Source: CAD feature listing. Evaluate the final solid. Frame: model axes, mm. A direction names the side the tool comes from. Give positions to 0.01 mm unless a question says otherwise; leave off trailing zeros. Order: outer loops, then holes, each group sorted by start corner. A loop starts at its lowest first (then second) coordinate and runs counter-clockwise, first axis right, second up.
from build123d import *

# Parameters (mm, degrees)
SKETCH1_W                = 58.5
SKETCH1_H                = 75
SKETCH1_R                = 8
SKETCH1_R_2              = 1.5
BOSS_EXTRUDE1_DEPTH      = 2.5
SKETCH4_W                = 58.5
SKETCH4_H                = 40
BOSS_EXTRUDE2_DEPTH      = 7.5
M3_CLEARANCE_HOLE1_D     = 3.2
M3_CLEARANCE_HOLE1_DEPTH = 4
M3_CLEARANCE_HOLE1_TIP   = 0.96137699
FILLET1_R                = 10
FILLET2_R                = 7.5


with BuildPart() as part:
    # Sketch1 → Boss-Extrude1 (new, symmetric)
    with BuildSketch(Plane.XY):
        with Locations((-9.25, 23)):
            Rectangle(SKETCH1_W, SKETCH1_H)
        Circle(SKETCH1_R, mode=Mode.SUBTRACT)
        with Locations((-24, -9)):
            Circle(SKETCH1_R_2, mode=Mode.SUBTRACT)
        with Locations((9, -9)):
            Circle(SKETCH1_R_2, mode=Mode.SUBTRACT)
        with Locations((9, 9)):
            Circle(SKETCH1_R_2, mode=Mode.SUBTRACT)
        with Locations((-24, 9)):
            Circle(SKETCH1_R_2, mode=Mode.SUBTRACT)
    extrude(amount=BOSS_EXTRUDE1_DEPTH, both=True)

    # Sketch4 → Boss-Extrude2 (add)
    with BuildSketch(Plane(origin=(0, 0, -2.5), x_dir=(-1, 0, 0), z_dir=(0, 0, -1))):
        with Locations((9.25, 40.5)):
            Rectangle(SKETCH4_W, SKETCH4_H)
    extrude(amount=BOSS_EXTRUDE2_DEPTH)

    # M3 Clearance Hole1
    with Locations(Plane(origin=(0, 60.5, 0), x_dir=(1, 0, 0), z_dir=(0, 1, 0))):
        with Locations((-31.95, 3), (11.75, 3)):
            Hole(M3_CLEARANCE_HOLE1_D / 2, depth=M3_CLEARANCE_HOLE1_DEPTH)
            with Locations((0, 0, -(M3_CLEARANCE_HOLE1_DEPTH + M3_CLEARANCE_HOLE1_TIP / 2))):  # 118° drill point
                Cone(0, M3_CLEARANCE_HOLE1_D / 2, M3_CLEARANCE_HOLE1_TIP, mode=Mode.SUBTRACT)

    # Fillet1
    fillet1_edges = [part.edges().sort_by_distance(p)[0] for p in [
        (20, -14.5, 0),
        (-38.5, -14.5, 0),
    ]]
    fillet(fillet1_edges, radius=FILLET1_R)

    # Fillet2
    fillet2_edges = [part.edges().sort_by_distance(p)[0] for p in [
        (-38.5, 40.5, -10),
        (20, 40.5, -10),
    ]]
    fillet(fillet2_edges, radius=FILLET2_R)


solid = part.part
1) Reachability of faces 1 (the face through (-9, 20.5, -6)), 2 (the face through (-9, 60.5, -4)), 3 (the face through (-30.35, 58.47, -3.07)) from +Z, -Z, +X, -X, +Y, -Y: full face, straight path, thin tool, end or side. Return the list, or none.
Checks:
face 1: -Z, +X, -X, -Y
face 2: +Z, -Z, +X, -X, +Y
face 3: +Y
2) Section query D-D on z = 0.5. Output: boundary loops of the cut face in (x, y), and give its area (3 significant figures).
Checks:
outline: (-38.5, -4.5) arc R10 ccw to (-28.5, -14.5) - (10, -14.5) arc R10 ccw to (20, -4.5) - (20, 60.5) - (-38.5, 60.5) - close; hole circle Ø3 at (-24, -9); hole circle Ø3 at (-24, 9); hole circle Ø16 at (0, 0); hole circle Ø3 at (9, -9); hole circle Ø3 at (9, 9)
area: 4,120 mm2
3) First-contact query: pin 1 Ø4 at (x, y) = (-11, 4) entering from -Z; pin 2 Ø4 at (x, z) = (-20.5, -6.5) entering from -Y; pin 3 Ø2 at (y, z) = (31, -7.5) entering from -X. Flat tips, straight axial feed; report the tip coordinate or a pass-through.
Checks:
pin 1: stops at z = -2.5
pin 2: stops at y = 20.5
pin 3: stops at x = -37.34
4) Pull-direction query (X, two-part tool) for faces 4 (the face through (-36.245, 40.78, -7.861)), 5 (the face through (-10, 3, -2.5)), 6 (the face through (11.529, 55.706, -2.831)), 7 (the face through (-25.2, 8.1, 0)); classes: +X half, -X half, draft (parallel to the pull), parting line (faces both ways), or undercut.
Checks:
face 4: -X half
face 5: draft
face 6: undercut
face 7: undercut
5) Ray query, L1, parallel to Y at x = 9, z = -0.4; L2, parallel to Y at x = 0, z = -1.4; L3, parallel to Y at x = 5.5, z = -6.75. Return the intervals inside material, ascending.
Checks:
L1: y = -14.5 to -10.5, -7.5 to 7.5, 10.5 to 60.5
L2: y = -14.5 to -8, 8 to 60.5
L3: y = 20.5 to 60.5
6) Section query B-B on x = -24. Output: boundary loops of the cut face in (y, z).
Checks:
outline: (-14.5, -2.5) - (-10.5, -2.5) - (-10.5, 2.5) - (-14.5, 2.5) - close; (-7.5, -2.5) - (7.5, -2.5) - (7.5, 2.5) - (-7.5, 2.5) - close; (10.5, -2.5) - (20.5, -2.5) - (20.5, -10) - (60.5, -10) - (60.5, 2.5) - (10.5, 2.5) - close
7) Section query A-A on y = 0. Output: boundary loops of the cut face in (x, z).
Checks:
outline: (-38.5, -2.5) - (-8, -2.5) - (-8, 2.5) - (-38.5, 2.5) - close; (8, -2.5) - (20, -2.5) - (20, 2.5) - (8, 2.5) - close
8) Section query C-C on x = 0. Output: boundary loops of the cut face in (y, z), and give its area (3 significant figures).
Checks:
outline: (-14.5, -2.5) - (-8, -2.5) - (-8, 2.5) - (-14.5, 2.5) - close; (8, -2.5) - (20.5, -2.5) - (20.5, -10) - (60.5, -10) - (60.5, 2.5) - (8, 2.5) - close
area: 595 mm2
